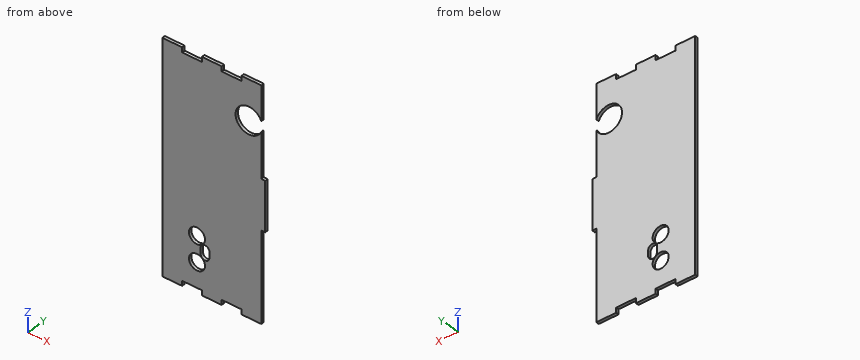
```python
from build123d import *

# Parameters (mm, degrees)
SKETCH1_R           = 8.1
BOSS_EXTRUDE1_DEPTH = 3


with BuildPart() as part:
    # Sketch1 → Boss-Extrude1 (new body)
    with BuildSketch(Plane(origin=(0, 0, 0), x_dir=(1, 0, 0), z_dir=(0, 1, 0))):
        with BuildLine():
            Line((-50, -111), (-50, -116))
            Line((-50, -116), (-30, -116))
            Line((-30, -116), (-30, -111))
            Line((-30, -111), (-10, -111))
            Line((-10, -111), (-10, -116))
            Line((-10, -116), (10, -116))
            Line((10, -116), (10, -111))
            Line((10, -111), (30, -111))
            Line((30, -111), (30, -116))
            Line((30, -116), (50, -116))
            Line((50, -116), (50, -111))
            Line((50, -111), (50, -81.099019514))
            ThreePointArc((50, -81.099019514), (24, -76), (50, -70.900980486))
            Line((50, -70.900980486), (50, -25))
            Line((50, -25), (54, -25))
            Line((54, -25), (54, 25))
            Line((54, 25), (50, 25))
            Line((50, 25), (50, 111))
            Line((50, 111), (50, 116))
            Line((50, 116), (30, 116))
            Line((30, 116), (30, 111))
            Line((30, 111), (10, 111))
            Line((10, 111), (10, 116))
            Line((10, 116), (-10, 116))
            Line((-10, 116), (-10, 111))
            Line((-10, 111), (-30, 111))
            Line((-30, 111), (-30, 116))
            Line((-30, 116), (-50, 116))
            Line((-50, 116), (-50, 111))
            Line((-50, 111), (-50, -111))
        make_face()
        with Locations(Location((-15, 60.4, 0), (0, 0, 270))):
            Circle(SKETCH1_R, mode=Mode.SUBTRACT)
        with Locations(Location((-15, 86, 0), (0, 0, 270))):
            Circle(SKETCH1_R, mode=Mode.SUBTRACT)
        with BuildLine():
            Line((-11.4, 70.35), (-11.4, 76.05))
            ThreePointArc((-11.4, 76.05), (-6.9, 80.55), (-2.4, 76.05))
            Line((-2.4, 76.05), (-2.4, 70.35))
            ThreePointArc((-2.4, 70.35), (-6.9, 65.85), (-11.4, 70.35))
        make_face(mode=Mode.SUBTRACT)
    extrude(amount=BOSS_EXTRUDE1_DEPTH)


solid = part.part
```
Part model, mm, in its own coordinate system. Give positions to 0.01 mm unless a question says otherwise; leave off trailing zeros. Order: outer loops, then holes, each group sorted by start corner. A loop starts at its lowest first (then second) coordinate and runs counter-clockwise, first axis right, second up. Notation, with made-up numbers: M 25.5,25.25 L 58.5,25.25 A24 ccw 58.5,63.25 Z; hole C 83,22 d9. An arc over 180 degrees is marked long. Use a Markdown table: item, result. Add a question column.
(1) Saw through at B-B, the plane x = 37.5. Give the cut face in (y, z).
(2) Saw through at D-D, the plane y = 1.45. Give the number of separate pieces and of enclosed holes in the cut face, and give its area (3 significant figures).
(3) Saw through at C-C, the plane x = -15. Give the cut face in (y, z), and give its area (3 significant figures).
(4) Saw through at A-A, the plane z = -60.4. Give the cut face in (x, y).
(5) Drop flat-ended pins along their axis: P1, Ø1.5, axis at y = 2, z = -61, coming from the +X side; P2, Ø0.9, axis at x = -18, y = 2, coming from the +Z side; P3, Ø14.5, axis at x = -15, z = -60.4, coming from the +Y side; P4, Ø1.5, axis at x = 20, y = 1, coming from the -Z side. Give the stop position or say it passes through.
(6) Probe line 1 along Z through (x, y) = (-15.5, 0.5); line 2 along Z through (x, y) = (37.5, 0.8); line 3 along Z through (x, y) = (-29, 1). List the from-to ranges inside material, lowest first. Write a range as [from, to].
Answer key:
| question | item | result |
|---|---|---|
| 1 | outline | M 0,-116 L 3,-116 L 3,62.5 L 0,62.5 Z; M 0,89.5 L 3,89.5 L 3,116 L 0,116 Z |
| 2 | separate pieces | 1 |
| 2 | enclosed holes | 3 |
| 2 | area | 21,900 mm^2 |
| 3 | outline | M 0,-111 L 3,-111 L 3,-94.1 L 0,-94.1 Z; M 0,-77.9 L 3,-77.9 L 3,-68.5 L 0,-68.5 Z; M 0,-52.3 L 3,-52.3 L 3,111 L 0,111 Z |
| 3 | area | 569 mm^2 |
| 4 | outline | M -50,0 L -23.1,0 L -23.1,3 L -50,3 Z; M -6.9,0 L 50,0 L 50,3 L -6.9,3 Z |
| 5 | P1 | x = 50 |
| 5 | P2 | z = 111 |
| 5 | P3 | through |
| 5 | P4 | z = -111 |
| 6 | line 1 | [-111, -94.08], [-77.92, -68.48], [-52.32, 111] |
| 6 | line 2 | [-116, 62.5], [89.5, 116] |
| 6 | line 3 | [-111, 111] |
